For this review, take the finished solid that the model builds, in its own axes (mm). A direction names the side the tool comes from. Give positions to 0.01 mm unless a question says otherwise; leave off trailing zeros. Loops run counter-clockwise (first coordinate to the right, second up) from the corner with the lowest first, then second, coordinate; pieces in that order, holes last.
```python
from build123d import *

# Parameters (mm, degrees)
SKETCH1_R                      = 4.05
BOSS_EXTRUDE1_DEPTH            = 7
FILLET1_R                      = 10
CBORE_FOR_M2_SHCS1_D           = 2.4
CBORE_FOR_M2_SHCS1_CBORE_D     = 4.4
CBORE_FOR_M2_SHCS1_CBORE_DEPTH = 2


with BuildPart() as part:
    # Sketch1 → Boss-Extrude1 (new body)
    with BuildSketch(Plane(origin=(0, 0, 0), x_dir=(0, 0, -1), z_dir=(1, 0, 0))):
        with BuildLine():
            ThreePointArc((-2.618193655, 12.222727273), (-15.499955296, 27.462773314), (-2.691546754, 42.764520172))
            ThreePointArc((-2.691546754, 42.764520172), (2.175410698, 49.715255756), (-4.775324886, 54.582213208))
            ThreePointArc((-4.775324886, 54.582213208), (-27.223172657, 31.392154992), (-12.172889367, 2.840909091))
            ThreePointArc((-12.172889367, 2.840909091), (-8.919155658, -8.757777249), (2.618193655, -12.222727273))
            ThreePointArc((2.618193655, -12.222727273), (15.499955296, -27.462773314), (2.691546754, -42.764520172))
            ThreePointArc((2.691546754, -42.764520172), (-2.175410698, -49.715255756), (4.775324886, -54.582213208))
            ThreePointArc((4.775324886, -54.582213208), (27.223172657, -31.392154992), (12.172889367, -2.840909091))
            ThreePointArc((12.172889367, -2.840909091), (8.919155658, 8.757777249), (-2.618193655, 12.222727273))
        make_face()
        Circle(SKETCH1_R, mode=Mode.SUBTRACT)
    extrude(amount=BOSS_EXTRUDE1_DEPTH)

    # Fillet1
    fillet1_edges = [part.edges().sort_by_distance(p)[0] for p in [
        (3.5, -2.840909091, -12.172889367),
        (3.5, -12.222727273, -2.618193655),
        (3.5, 2.840909091, 12.172889367),
        (3.5, 12.222727273, 2.618193655),
    ]]
    fillet(fillet1_edges, radius=FILLET1_R)

    # CBORE for M2 SHCS1 (through all)
    with Locations(Plane(origin=(7, 0, 0), x_dir=(0, 0, -1), z_dir=(1, 0, 0))):
        with Locations((-5.656854249, 5.656854249), (0, 8), (5.656854249, 5.656854249), (8, 0), (5.656854249, -5.656854249), (0, -8), (-5.656854249, -5.656854249), (-8, 0)):
            CounterBoreHole(CBORE_FOR_M2_SHCS1_D / 2, CBORE_FOR_M2_SHCS1_CBORE_D / 2, CBORE_FOR_M2_SHCS1_CBORE_DEPTH)


solid = part.part
```
Item 1: Take a section at D-D on z = 21. Give the boundary of the cut face in (x, y), and give its area (3 significant figures).
Answer:
outline: (0, 9.74) - (7, 9.74) - (7, 45.26) - (0, 45.26) - close
area: 249 mm2
Item 2: Tool access review of faces 4 (the cylindrical face through (6.014, 5.754, 7.855)), 5 (the cylindrical face through (2.46, -5.6, 4.46)): name each direction out of +Z, -Z, +X, -X, +Y, -Y from which nothing blocks a thin tool from reaching the whole face with its end or side.
Answer:
face 4: +X
face 5: +X, -X
Item 3: The part is to be moulded in two halves that separate along Y. For faces 1 (the flat face through (7, -4, -2)), 2 (the cylindrical face through (6.014, 6.318, -7.755)), 3 (the cylindrical face through (3.451, 34.257, 26.657)), say which applies: released by +Y, released by -Y, zero draft, split by the parting line, or undercut.
Answer:
face 1: zero draft
face 2: undercut
face 3: split by the parting line
Item 4: Clearance check with flat-ended pins moving along their axes: pin 1 Ø3 at (x, y) = (3.5, -2.5) entering from -Z; pin 2 Ø3 at (y, z) = (8, 0) entering from +X; pin 3 Ø3 at (x, y) = (4.5, 31.5) entering from -Z. State where each tip first meets the part, or that it passes through.
Answer:
pin 1: stops at z = -14.85
pin 2: stops at x = 5
pin 3: stops at z = 14.49
Item 5: For L1, parallel to Y at x = 4.5, z = -8.5; L2, parallel to Z at x = 5.25, y = -4.5; L3, parallel to Y at x = 2, z = 0, list the stretches that pass through material, from the lowest coordinate up.
Answer:
L1: y = -53.65 to -40.46, -14.54 to -1.09, 1.09 to 9.17
L2: z = -15.32 to -7.53, -3.79 to 3.79, 7.53 to 11.66
L3: y = -53.37 to -43.98, -12.5 to -9.2, -6.8 to -4.05, 4.05 to 6.8, 9.2 to 12.5, 43.98 to 53.37
Item 6: Take a section at A-A on z = 0. State how many separate pieces and enclosed holes the cut face has, and give its area (3 significant figures).
Answer:
separate pieces: 6
enclosed holes: 0
area: 208 mm2
